The figure shows three views and two pictorial views of one solid part (mm, origin at its lowest corner). Answer the questions. A direction names the side the tool comes from. Coordinates: 2 decimals unless noted, no trailing zeros. Write each loop counter-clockwise with the first axis right and the second up, starting at its lowest first coordinate (ties: lowest second). Pieces come first, ordered by that corner, then holes.
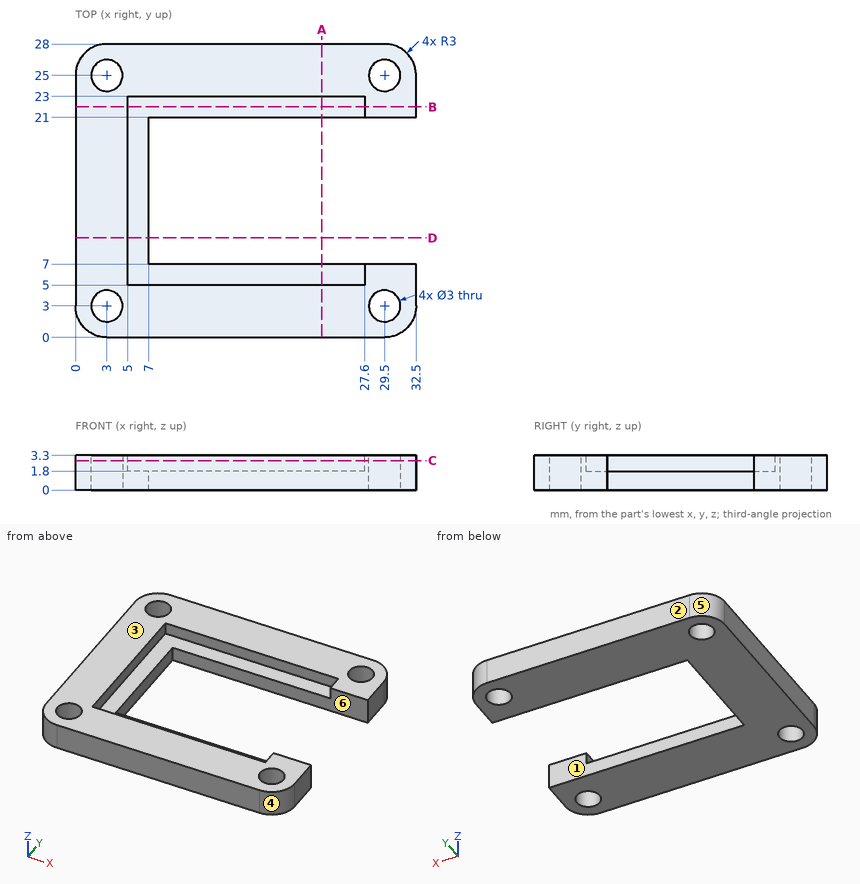
Q1. The part is cut by section C-C, the plane z = 2.8. Write down the section's boundary in (x, y), then the cut area to 3 significant figures.
Answers below:
outline: (0, 3) arc R3 ccw to (3, 0) - (29.5, 0) arc R3 ccw to (32.5, 3) - (32.5, 7) - (27.6, 7) - (27.6, 5) - (5, 5) - (5, 23) - (27.6, 23) - (27.6, 21) - (32.5, 21) - (32.5, 25) arc R3 ccw to (29.5, 28) - (3, 28) arc R3 ccw to (0, 25) - close; hole circle Ø3 at (3, 3); hole circle Ø3 at (3, 25); hole circle Ø3 at (29.5, 3); hole circle Ø3 at (29.5, 25)
area: 399 mm2
Q2. Find the intervals of material crossed by probe 1 along Y at (x, z) = (3, 1.75); probe 2 along Y at (x, z) = (23.5, 2.7); probe 3 along Y at (x, z) = (29.5, 2.2), in increasing order.
Answers below:
probe 1: y = 0 to 1.5, 4.5 to 23.5, 26.5 to 28
probe 2: y = 0 to 5, 23 to 28
probe 3: y = 0 to 1.5, 4.5 to 7, 21 to 23.5, 26.5 to 28
Q3. Given pin 1 (0.7 mm diameter, centred on y = 6.5, z = 2.5, fed in from -X); pin 2 (1.6 mm diameter, centred on y = 14, z = 2.5, fed in from +X); pin 3 (2.5 mm diameter, centred on x = 29.5, y = 25, fed in from -Z); pin 4 (10 mm diameter, centred on x = 13.5, y = 11, fed in from +Z), each flat-ended and moving along its own axis, determine where each tip first touches the part or whether it passes through.
Answers below:
pin 1: stops at x = 0
pin 2: stops at x = 7
pin 3: passes through
pin 4: stops at z = 1.8
Q4. The part is cut by section B-B, the plane y = 22. Write down the section's boundary in (x, z), then the cut area to 4 significant figures.
Answers below:
outline: (0, 0) - (32.5, 0) - (32.5, 3.3) - (27.6, 3.3) - (27.6, 1.8) - (5, 1.8) - (5, 3.3) - (0, 3.3) - close
area: 73.35 mm2
Q5. The part is cut by section D-D, the plane y = 9.5. Write down the section's boundary in (x, z), then the cut area to 3 significant figures.
Answers below:
outline: (0, 0) - (7, 0) - (7, 1.8) - (5, 1.8) - (5, 3.3) - (0, 3.3) - close
area: 20.1 mm2
Q6. Determine the mould class of the marked faces 1, 2, 3 and 4 for opening direction Y: released by +Y, released by -Y, zero draft, split by the parting line, or undercut.
Answers below:
face 1: undercut
face 2: released by +Y
face 3: zero draft
face 4: released by -Y
Q7. Which of the six approach directions +Z, -Z, +X, -X, +Y, -Y give full straight-line access (tool end or side, diameter ignored) to the marked faces 5 and 6?
Answers below:
face 5: +Z, -Z, -X, +Y
face 6: +Z, -Z, +X
Q8. The part is cut by section A-A, the plane x = 23.5. Write down the section's boundary in (y, z).
Answers below:
outline: (0, 0) - (7, 0) - (7, 1.8) - (5, 1.8) - (5, 3.3) - (0, 3.3) - close; (21, 0) - (28, 0) - (28, 3.3) - (23, 3.3) - (23, 1.8) - (21, 1.8) - close
